Source: CAD feature listing. Evaluate the final solid. Frame: model axes, mm. Give positions to 0.01 mm unless a question says otherwise; leave off trailing zeros. Order: outer loops, then holes, each group sorted by start corner. A loop starts at its lowest first (then second) coordinate and runs counter-clockwise, first axis right, second up. Notation, with made-up numbers: M -33.75,22.5 L -24.75,22.5 A15 cw -24.75,49.5 Z; hole C 18,45 d1. An arc over 180 degrees is marked long. Answer as a JSON object with one key per item and string values. Group by question number.
1. Material intervals for L1, parallel to X at y = 0.2, z = 2.25; L2, parallel to Z at x = -30, y = 0.75; L3, parallel to Z at x = -27.5, y = 0.3, sorted ascending. Write a range as [from, to].
2. Section query A-A (y = 0.8). Output: boundary loops of the cut face in (x, z).
3. Section query C-C (z = -5.25). Output: boundary loops of the cut face in (x, y), plus the area to 3 significant figures.
4. Pin query (flat end, axial travel): P1, Ø0.5, axis at y = 0.5, z = 1.5, coming from the -X side; P2, Ø0.5, axis at y = 0.5, z = 1.5, coming from the +X side. Return the tip coordinate at first contact, or that it passes through.
5. Section query B-B (x = -6.5). Output: boundary loops of the cut face in (y, z), plus the area to 3 significant figures.
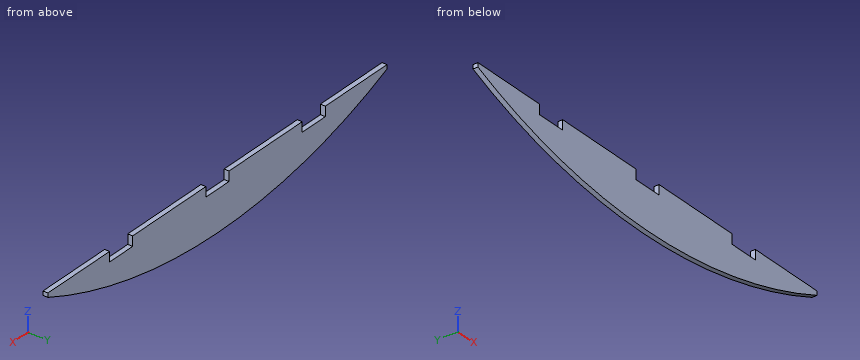
from build123d import *

# Parameters (mm, degrees)
EXTRUDE_1_DEPTH     = 1
SKETCH_2_W          = 6
SKETCH_2_H          = 4
CUT_EXTRUDE_1_DEPTH = 2


with BuildPart() as part:
    # 草图1 → 凸台-拉伸1 (new body)
    with BuildSketch(Plane(origin=(0, 0, 0), x_dir=(1, 0, 0), z_dir=(0, 1, 0))):
        with BuildLine():
            Line((-30, -3), (-44, -3))
            Line((-44, -3), (-44, -2.158291102))
            ThreePointArc((-44, -2.158291102), (0, 7.280007457), (44, -2.158291102))
            Line((44, -2.158291102), (44, -3))
            Line((44, -3), (30, -3))
            Line((30, -3), (-30, -3))
        make_face()
    extrude(amount=EXTRUDE_1_DEPTH)

    # 草图2 → 切除-拉伸1 (cut, through all)
    with BuildSketch(Plane.XZ):
        with Locations((0, 3)):
            Rectangle(SKETCH_2_W, SKETCH_2_H)
        with Locations((25, 3)):
            Rectangle(SKETCH_2_W, SKETCH_2_H)
        with Locations((-25, 3)):
            Rectangle(SKETCH_2_W, SKETCH_2_H)
    extrude(amount=-CUT_EXTRUDE_1_DEPTH, mode=Mode.SUBTRACT)


solid = part.part
Answer sheet:
{
 "1": {"L1": "[-44, -28], [-22, -3], [3, 22], [28, 44]", "L2": "[-3, 3]", "L3": "[-3.7, 1]"},
 "2": {"outline": "M -44,2.16 A107.28 ccw 44,2.16 L 44,3 L 28,3 L 28,1 L 22,1 L 22,3 L 3,3 L 3,1 L -3,1 L -3,3 L -22,3 L -22,1 L -28,1 L -28,3 L -44,3 Z"},
 "3": {"outline": "M -20.77,0 L 20.77,0 L 20.77,1 L -20.77,1 Z", "area": "41.5 mm^2"},
 "4": {"P1": "x = -43.08", "P2": "x = 43.08"},
 "5": {"outline": "M 0,-7.08 L 1,-7.08 L 1,3 L 0,3 Z", "area": "10.1 mm^2"}
}
